Design review of the part built by this model. Coordinates are the model's own, in mm. A direction names the side the tool comes from. Give positions to 0.01 mm unless a question says otherwise; leave off trailing zeros. Order: outer loops, then holes, each group sorted by start corner. A loop starts at its lowest first (then second) coordinate and runs counter-clockwise, first axis right, second up. Notation, with made-up numbers: (-32.75, -21.75) -> (-14.75, -21.75) arc R26 ccw to (-14.75, 13.25) -> close; hole circle Ø4 at (-34.5, -20). An arc over 180 degrees is marked (long way). Return JSON: item names as keys, results as strings.
```python
from build123d import *

# Parameters (mm, degrees)
F0_W          = 25
F0_H          = 10
F1_DEPTH      = 6
F2_W          = 5
F2_H          = 10
F3_DEPTH      = 10
F4_R          = 1.25
F5_DEPTH      = 6.001
F6_R          = 4.99999
F7_R          = 1.6
F8_DEPTH      = 15.001
F9_R          = 1
F10_T1_DEPTH  = 8
F10_T6_ANGLE  = 233.435380504
F10_T11_ANGLE = 233.435380504
F10_T16_ANGLE = 233.435380504
F10_T21_ANGLE = 233.435380504


# Not quite as in the source:
# - a fillet or chamfer that OpenCascade refuses, or shapes differently, is made with other operations: its cross-section is extruded or revolved along the edge and cut away or added
# - a fillet or chamfer is up to 0.001 mm smaller than in the source, because OpenCascade refuses the exact size
# - a pattern or mirror of a feature is missing from the dataset's text; its kind, count and spacing are read off the source's solid


with BuildPart() as f1:
    # F0 (on Top) → F1 (new body)
    with BuildSketch(Plane.XY):
        Rectangle(F0_W, F0_H)
    extrude(amount=F1_DEPTH)

    # F2 (on face) → F3 (join)
    with BuildSketch(Plane.XY.offset(6)):
        Rectangle(F2_W, F2_H)
    extrude(amount=F3_DEPTH)

    # F4 (on face) → F5 (cut, through all)
    with BuildSketch(Plane.XY.offset(6)):
        with Locations((-7.5, 0)):
            Circle(F4_R)
    f5 = extrude(amount=-F5_DEPTH, mode=Mode.SUBTRACT)

    # F5_copies: F5 across plane
    add(f5.mirror(Plane(origin=(0, 0, 0), x_dir=(0, 0, 1), z_dir=(1, 0, 0))), mode=Mode.SUBTRACT)

    # F6 (radius 5 in the source; OpenCascade refuses exactly that, so slightly less here)
    f6_edges = [f1.edges().sort_by_distance(p)[0] for p in [
        (0, -5, 16),
        (0, 5, 16),
    ]]
    fillet(f6_edges, radius=F6_R)

    # F7 (on face) → F8 (cut, through all)
    with BuildSketch(Plane(origin=(-2.5, 0, 0), x_dir=(0, -1, 0), z_dir=(-1, 0, 0))):
        with Locations((0, 11)):
            Circle(F7_R)
    extrude(amount=-F8_DEPTH, mode=Mode.SUBTRACT)

    # F9
    f9_edges = [f1.edges().sort_by_distance(p)[0] for p in [
        (7.5, -5, 6),
        (12.5, 0, 6),
        (7.5, 5, 6),
        (12.5, -5, 3),
        (12.5, 5, 3),
        (-12.5, -5, 3),
        (-12.5, 5, 3),
        (-12.5, 0, 6),
        (-7.5, -5, 6),
        (-7.5, 5, 6),
    ]]
    fillet(f9_edges, radius=F9_R)

    # F10: fillet of radius 1 on 2 edges, made by hand

    # F10_s2 → F10_t1 (join)
    with BuildSketch(Plane.XZ.offset(-4)):
        with BuildLine():
            ThreePointArc((2.4996, 7.0009656854), (2.7928932188, 6.2928932188), (3.5009656854, 5.9996))
            Line((3.5009656854, 5.9996), (3.5009656854, 5.8994634315))
            ThreePointArc((3.5009656854, 5.8994634315), (3.0004828427, 5.8998634315), (2.5, 5.8998634315))
            Line((2.5, 5.8998634315), (2.3998634315, 6))
            ThreePointArc((2.3998634315, 6), (2.3998634315, 6.5004828427), (2.3994634315, 7.0009656854))
            Line((2.3994634315, 7.0009656854), (2.4996, 7.0009656854))
        make_face()
        with BuildLine():
            ThreePointArc((-2.4996, 7.0009656854), (-2.7928932188, 6.2928932188), (-3.5009656854, 5.9996))
            Line((-3.5009656854, 5.9996), (-3.5009656854, 5.8994634315))
            ThreePointArc((-3.5009656854, 5.8994634315), (-3.0004828427, 5.8998634315), (-2.5, 5.8998634315))
            Line((-2.5, 5.8998634315), (-2.3998634315, 6))
            ThreePointArc((-2.3998634315, 6), (-2.3998634315, 6.5004828427), (-2.3994634315, 7.0009656854))
            Line((-2.3994634315, 7.0009656854), (-2.4996, 7.0009656854))
        make_face()
    extrude(amount=F10_T1_DEPTH)


with BuildPart() as f10_tool4:
    # F10_s5 → F10_t6 (revolve)
    with BuildSketch(Plane.XZ.offset(-4)):
        with BuildLine():
            ThreePointArc((-2.4996, 7.0009656854), (-2.7928932188, 6.2928932188), (-3.5009656854, 5.9996))
            Line((-3.5009656854, 5.9996), (-3.5009656854, 5.8994634315))
            ThreePointArc((-3.5009656854, 5.8994634315), (-3.0004828427, 5.8998634315), (-2.5, 5.8998634315))
            Line((-2.5, 5.8998634315), (-2.3998634315, 6))
            ThreePointArc((-2.3998634315, 6), (-2.3998634315, 6.5004828427), (-2.3994634315, 7.0009656854))
            Line((-2.3994634315, 7.0009656854), (-2.4996, 7.0009656854))
        make_face()
    revolve(axis=Axis((-2.5, 4, 5), (-1, 0, 0)), revolution_arc=F10_T6_ANGLE)

    split(bisect_by=Plane.XZ.offset(-5), keep=Keep.TOP)


with BuildPart() as f1_1:
    add(f1.part)

    # F10_t3: union F10_tool4
    add(f10_tool4.part)


with BuildPart() as f10_tool9:
    # F10_s10 → F10_t11 (revolve)
    with BuildSketch(Plane(origin=(0, 0.9728322798, 1.3116110753), x_dir=(1, 0, 0), z_dir=(0, 0.5957290165, 0.8031854947))):
        with BuildLine():
            ThreePointArc((-3.5009656854, -5.1917870613), (-2.7928932188, -4.8984938425), (-2.4996, -4.1904213759))
            Line((-2.4996, -4.1904213759), (-2.3994634315, -4.1904213759))
            ThreePointArc((-2.3994634315, -4.1904213759), (-2.3998634315, -4.6909042186), (-2.3998634315, -5.1913870613))
            Line((-2.3998634315, -5.1913870613), (-2.5, -5.2915236298))
            ThreePointArc((-2.5, -5.2915236298), (-3.0004828427, -5.2915236298), (-3.5009656854, -5.2919236298))
            Line((-3.5009656854, -5.2919236298), (-3.5009656854, -5.1917870613))
        make_face()
    revolve(axis=Axis((-2.5, -4, 5), (-1, 0, 0)), revolution_arc=F10_T11_ANGLE)

    split(bisect_by=Plane.XZ.offset(5), keep=Keep.BOTTOM)


with BuildPart() as f1_2:
    add(f1_1.part)

    # F10_t8: union F10_tool9
    add(f10_tool9.part)


with BuildPart() as f10_tool14:
    # F10_s15 → F10_t16 (revolve)
    with BuildSketch(Plane(origin=(0, 0.9728322798, 1.3116110753), x_dir=(1, 0, 0), z_dir=(0, 0.5957290165, 0.8031854947))):
        with BuildLine():
            ThreePointArc((3.5009656854, -5.1917870613), (2.7928932188, -4.8984938425), (2.4996, -4.1904213759))
            Line((2.4996, -4.1904213759), (2.3994634315, -4.1904213759))
            ThreePointArc((2.3994634315, -4.1904213759), (2.3998634315, -4.6909042186), (2.3998634315, -5.1913870613))
            Line((2.3998634315, -5.1913870613), (2.5, -5.2915236298))
            ThreePointArc((2.5, -5.2915236298), (3.0004828427, -5.2915236298), (3.5009656854, -5.2919236298))
            Line((3.5009656854, -5.2919236298), (3.5009656854, -5.1917870613))
        make_face()
    revolve(axis=Axis((2.5, -4, 5), (-1, 0, 0)), revolution_arc=F10_T16_ANGLE)

    split(bisect_by=Plane.XZ.offset(5), keep=Keep.BOTTOM)


with BuildPart() as f1_3:
    add(f1_2.part)

    # F10_t13: union F10_tool14
    add(f10_tool14.part)


with BuildPart() as f10_tool19:
    # F10_s20 → F10_t21 (revolve)
    with BuildSketch(Plane.XZ.offset(-4)):
        with BuildLine():
            ThreePointArc((2.4996, 7.0009656854), (2.7928932188, 6.2928932188), (3.5009656854, 5.9996))
            Line((3.5009656854, 5.9996), (3.5009656854, 5.8994634315))
            ThreePointArc((3.5009656854, 5.8994634315), (3.0004828427, 5.8998634315), (2.5, 5.8998634315))
            Line((2.5, 5.8998634315), (2.3998634315, 6))
            ThreePointArc((2.3998634315, 6), (2.3998634315, 6.5004828427), (2.3994634315, 7.0009656854))
            Line((2.3994634315, 7.0009656854), (2.4996, 7.0009656854))
        make_face()
    revolve(axis=Axis((2.5, 4, 5), (-1, 0, 0)), revolution_arc=F10_T21_ANGLE)

    split(bisect_by=Plane.XZ.offset(-5), keep=Keep.TOP)


with BuildPart() as f1_4:
    add(f1_3.part)

    # F10_t18: union F10_tool19
    add(f10_tool19.part)


solid = f1_4.part
```
Item 1: For pin 1 (3 mm diameter, centred on x = -7.5, y = 0, fed in from -Z); pin 2 (2 mm diameter, centred on x = 0, z = 14, fed in from -Y); pin 3 (3 mm diameter, centred on y = -1, z = 11.5, fed in from +X); pin 4 (3 mm diameter, centred on y = 1.5, z = 12, fed in from -X), all flat-tipped, find the tip position at first contact; note any pin that passes through.
Result set:
{"pin 1": "stops at z = 0", "pin 2": "stops at y = -4.58", "pin 3": "stops at x = 2.5", "pin 4": "stops at x = -2.5"}
Item 2: Machinability: for faces 5 (the face through (-7.43, -4.715, 5.699)), 6 (the face through (-2.5, 0, 9)), 7 (the face through (7.543, 4.699, 5.715)), 8 (the face through (7.543, -4.715, 5.699)), which of the approach directions +Z, -Z, +X, -X, +Y, -Y give a long, thin tool a straight path to every point of the face, cutting with its end or side? Answer none if there is none.
Result set:
{"face 5": "+Z, -X, -Y", "face 6": "+Z, -X, +Y, -Y", "face 7": "+Z, +X, +Y", "face 8": "+Z, +X, -Y"}
Item 3: Add section B-B (x = -7.5). Give the boundary of the cut face in (y, z), plus the area to 3 significant figures.
Result set:
{"outline": "(-5, 0) -> (-1.25, 0) -> (-1.25, 6) -> (-4, 6) arc R1 ccw to (-5, 5) -> close; (1.25, 0) -> (5, 0) -> (5, 5) arc R1 ccw to (4, 6) -> (1.25, 6) -> close", "area": "44.6 mm^2"}
Item 4: Mouldability with a two-part tool opening along Z and no side actions: class faces 1 (the face through (-0.04, 0.35, 9.44)), 2 (the face through (-12.215, 4.699, 2.535)), 3 (the face through (-2.785, 0.056, 6.3)), 4 (the face through (0, 0, 0)) as released by +Z, released by -Z, zero draft, split by the parting line, or undercut.
Result set:
{"face 1": "undercut", "face 2": "zero draft", "face 3": "released by +Z", "face 4": "released by -Z"}
Item 5: Add section A-A (z = 3.25). Give the boundary of the cut face in (x, y), plus the area to 3 significant figures.
Result set:
{"outline": "(-12.5, -4) arc R1 ccw to (-11.5, -5) -> (11.5, -5) arc R1 ccw to (12.5, -4) -> (12.5, 4) arc R1 ccw to (11.5, 5) -> (-11.5, 5) arc R1 ccw to (-12.5, 4) -> close; hole circle Ø2.5 at (-7.5, 0); hole circle Ø2.5 at (7.5, 0)", "area": "239 mm^2"}
Item 6: Wall thickness on L1, parallel to X at y = 0.75, z = 2.75; L2, parallel to X at y = -0.5, z = 4; L3, parallel to Y at x = -7.5, z = 4.35: over which ranges is each line inside the solid? List them lowest first. Write a range as [from, to].
Result set:
{"L1": "x = [-12.5, -8.5], [-6.5, 6.5], [8.5, 12.5]", "L2": "x = [-12.5, -8.65], [-6.35, 6.35], [8.65, 12.5]", "L3": "y = [-5, -1.25], [1.25, 5]"}
Item 7: Add section D-D (y = -2.5). Give the boundary of the cut face in (x, z), plus the area to 3 significant figures.
Result set:
{"outline": "(-12.5, 0) -> (12.5, 0) -> (12.5, 5) arc R1 ccw to (11.5, 6) -> (3.47, 6) arc R1 cw to (2.5, 6.97) -> (2.5, 15.33) -> (-2.5, 15.33) -> (-2.5, 6.97) arc R1 cw to (-3.47, 6) -> (-11.5, 6) arc R1 ccw to (-12.5, 5) -> close", "area": "197 mm^2"}
